Part model, mm, in its own coordinate system. Give positions to 0.01 mm unless a question says otherwise; leave off trailing zeros. Order: outer loops, then holes, each group sorted by start corner. A loop starts at its lowest first (then second) coordinate and runs counter-clockwise, first axis right, second up. Notation, with made-up numbers: M 31.25,-3 L 50.25,-3 A18 cw 50.25,6 Z; hole C -27,80 d8. An arc over 180 degrees is marked long. Return JSON: item names as keys, results as strings.
from build123d import *

# Parameters (mm, degrees)
SKETCH1_R           = 2.6
BOSS_EXTRUDE1_DEPTH = 3
CHAMFER1_SIZE       = 0.5


with BuildPart() as part:
    # Sketch1 → Boss-Extrude1 (new, symmetric)
    with BuildSketch(Plane(origin=(0, 0, 0), x_dir=(1, 0, 0), z_dir=(0, 1, 0))):
        with BuildLine():
            Line((0, -7.5), (120, -7.5))
            ThreePointArc((120, -7.5), (127.5, 0), (120, 7.5))
            Line((120, 7.5), (0, 7.5))
            ThreePointArc((0, 7.5), (-7.5, 0), (0, -7.5))
        make_face()
        with Locations(Location((0, 0, 0), (0, 0, 270))):
            Circle(SKETCH1_R, mode=Mode.SUBTRACT)
        with Locations(Location((120, 0, 0), (0, 0, 270))):
            Circle(SKETCH1_R, mode=Mode.SUBTRACT)
    extrude(amount=BOSS_EXTRUDE1_DEPTH, both=True)

    # Chamfer1
    chamfer1_edges = [part.edges().sort_by_distance(p)[0] for p in [
        (120, -3, -2.6),
        (0, -3, -2.6),
        (120, 3, -2.6),
        (60, 3, 7.5),
        (127.5, 3, 0),
        (60, 3, -7.5),
        (-7.5, 3, 0),
        (0, 3, -2.6),
        (-7.5, -3, 0),
        (60, -3, -7.5),
        (127.5, -3, 0),
        (60, -3, 7.5),
    ]]
    chamfer(chamfer1_edges, length=CHAMFER1_SIZE)


solid = part.part
Q1. Band-saw the part on A-A (z = 0). Give the cut face in (x, y).
Established:
{"outline": "M -7.5,-2.5 L -7,-3 L -3.1,-3 L -2.6,-2.5 L -2.6,2.5 L -3.1,3 L -7,3 L -7.5,2.5 Z; M 2.6,-2.5 L 3.1,-3 L 116.9,-3 L 117.4,-2.5 L 117.4,2.5 L 116.9,3 L 3.1,3 L 2.6,2.5 Z; M 122.6,-2.5 L 123.1,-3 L 127,-3 L 127.5,-2.5 L 127.5,2.5 L 127,3 L 123.1,3 L 122.6,2.5 Z"}
Q2. Probe line 1 along X through (y, z) = (1.55, 0); line 2 along X through (y, z) = (0.5, -1); line 3 along X through (y, z) = (0, 5.25). List the from-to ranges inside material, lowest first.
Established:
{"line 1": "x = -7.5 to -2.6, 2.6 to 117.4, 122.6 to 127.5", "line 2": "x = -7.43 to -2.4, 2.4 to 117.6, 122.4 to 127.43", "line 3": "x = -5.36 to 125.36"}
Q3. Band-saw the part on B-B (y = -0.75). Give the cut face in (x, z), then the cut area to 3 significant figures.
Established:
{"outline": "M 0,-7.5 L 120,-7.5 A7.5 ccw 120,7.5 L 0,7.5 A7.5 ccw Z; hole C 0,0 d5.2; hole C 120,0 d5.2", "area": "1,930 mm²"}
Q4. Two-plate mould, pull along Z, no slides. Class faces 1 (the flat face through (61, 0, -7.5)), 2 (the cylindrical face through (0.78, -0.04, 2.48)), 3 (the conical face through (-7.134, -2.865, -0.157)): +Z half, -Z half, draft (parallel to the pull), parting line (faces both ways), or undercut.
Established:
{"face 1": "-Z half", "face 2": "undercut", "face 3": "parting line"}
Q5. Pin check, flat tips, straight feed: pin 1 (4.5 mm diameter, centred on x = 0, z = 0, fed in from +Y); pin 2 (1 mm diameter, centred on y = 2.5, z = -3.5, fed in from +X). Stop position of each tip, or through.
Established:
{"pin 1": "passes through", "pin 2": "stops at x = 126.87"}
